Can you work these out from the drawing? Everything is in mm from the part's minimum corner. A direction names the side the tool comes from. Coordinates: 2 decimals unless noted, no trailing zeros. Loops run counter-clockwise (first coordinate to the right, second up) from the corner with the lowest first, then second, coordinate; pieces in that order, holes last. Notation, with made-up numbers: (-22, 12) - (11, 12) arc R23 ccw to (11, 43) - close; hole circle Ø4 at (0.5, 17.25). An arc over 180 degrees is marked (long way). Put each result on its own line as item: value. Start each with the question number.
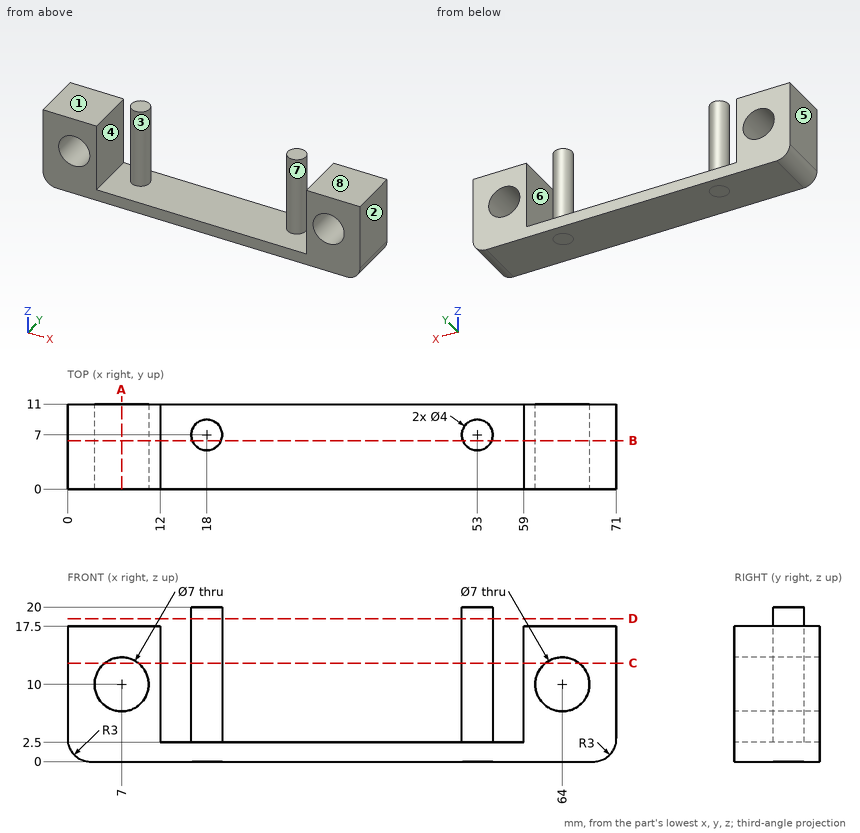
(1) If we mould it in two halves opening along X, with no side actions, what happens to the marked faces 5, 6, 7 and 8? For each: pulls with the +X half, pulls with the -X half, needs draft (parallel to the pull), parting line crosses it, or undercut.
(2) I need wall thicknesses on L1, parallel to X at y = 7, z = 3.25; L2, parallel to X at y = 10, z = 5.75; L3, parallel to Z at x = 64, y = 7.25. Which ranges of each line are inside material? Lowest first, please. Write a range as [from, to].
(3) I want a section at B-B on y = 6.25. List the corners of the cut face in (x, z) for me.
(4) I want a section at D-D on z = 18.5. List the corners of the cut face in (x, y) for me, and give its area (3 significant figures).
(5) I want a section at A-A on x = 7. List the corners of the cut face in (y, z) for me.
(6) For pin 1 Ø5.5 at (x, y) = (37.5, 5.5) entering from +Z; pin 2 Ø5 at (x, y) = (62.5, 4.5) entering from +Z, each with a flat end and sliding along its axis, tell me the tip position at first contact or that it passes through.
(7) Which directions (+Z, -Z, +X, -X, +Y, -Y) give clear straight access to the entire face, cutting with the end or side of a thin tool? Please do the marked faces 1, 2, 3 and 4.
(8) I want a section at C-C on z = 12.75. List the corners of the cut face in (x, y) for me, and give its area (3 significant figures).
Answer sheet:
1. face 5: pulls with the -X half
1. face 6: undercut
1. face 7: undercut
1. face 8: needs draft
2. L1: x = [0, 12], [16, 20], [51, 55], [59, 71]
2. L2: x = [0, 12], [59, 71]
2. L3: z = [0, 6.5], [13.5, 17.5]
3. outline: (0, 3) arc R3 ccw to (3, 0) - (16.15, 0) - (51.15, 0) - (68, 0) arc R3 ccw to (71, 3) - (71, 17.5) - (59, 17.5) - (59, 2.5) - (54.85, 2.5) - (54.85, 20) - (51.15, 20) - (51.15, 2.5) - (19.85, 2.5) - (19.85, 20) - (16.15, 20) - (16.15, 2.5) - (12, 2.5) - (12, 17.5) - (0, 17.5) - close; hole circle Ø7 at (7, 10); hole circle Ø7 at (64, 10)
4. outline: circle Ø4 at (18, 7); circle Ø4 at (53, 7)
4. area: 25.1 mm^2
5. outline: (0, 0) - (11, 0) - (11, 6.5) - (0, 6.5) - close; (0, 13.5) - (11, 13.5) - (11, 17.5) - (0, 17.5) - close
6. pin 1: stops at z = 2.5
6. pin 2: stops at z = 17.5
7. face 1: +Z, -X, +Y, -Y
7. face 2: +Z, -Z, +X, +Y, -Y
7. face 3: +Z
7. face 4: +Z, +Y, -Y
8. outline: (0, 0) - (4.83, 0) - (4.83, 11) - (0, 11) - close; (9.17, 0) - (12, 0) - (12, 11) - (9.17, 11) - close; circle Ø4 at (18, 7); circle Ø4 at (53, 7); (59, 0) - (61.83, 0) - (61.83, 11) - (59, 11) - close; (66.17, 0) - (71, 0) - (71, 11) - (66.17, 11) - close
8. area: 194 mm^2
